```python
from build123d import *

# Parameters (mm, degrees)
CHANFREIN1_SIZE         = 0.5
CHANFREIN2_SIZE         = 1
ESQUISSE2_W             = 9
ESQUISSE2_H             = 30
ENL_V_MAT_EXTRU_1_DEPTH = 30
ENL_V_MAT_EXTRU_2_REACH = 84.195
ESQUISSE3_R             = 4.1
CHANFREIN3_SIZE         = 0.5
ENL_V_MAT_EXTRU_3_REACH = 53.962
ESQUISSE5_W             = 20
ESQUISSE5_H             = 3.5


with BuildPart() as part:
    # Esquisse1 → Révolution1 (revolve)
    with BuildSketch(Plane.XY, mode=Mode.PRIVATE) as r_volution1_sk:
        Polygon((-50, 8), (-65, 8), (-65, 5), (-66, 5), (-66, 6), (-80, 6), (-80, 0), (0, 0), (0, 10), (-50, 10), align=None)
    revolve(r_volution1_sk.sketch.rotate(Axis((0, 0, 0), (1, 0, 0)), 90), axis=Axis((0, 0, 0), (1, 0, 0)))

    # Chanfrein1
    chanfrein1_edges = [part.edges().sort_by_distance(p)[0] for p in [
        (-50, 0, -10),
        (0, 0, -10),
        (-65, 0, -8),
    ]]
    chamfer(chanfrein1_edges, length=CHANFREIN1_SIZE)

    # Chanfrein2
    chanfrein2_edges = [part.edges().sort_by_distance(p)[0] for p in [
        (-80, 0, -6),
    ]]
    chamfer(chanfrein2_edges, length=CHANFREIN2_SIZE)

    # Esquisse2 → Enlèv. mat.-Extru.1 (cut)
    with BuildSketch(Plane(origin=(0, 0, 0), x_dir=(0, 0, -1), z_dir=(1, 0, 0))):
        with Locations((-10.5, 0)):
            Rectangle(ESQUISSE2_W, ESQUISSE2_H)
        with Locations((10.5, 0)):
            Rectangle(ESQUISSE2_W, ESQUISSE2_H)
    extrude(amount=-ENL_V_MAT_EXTRU_1_DEPTH, mode=Mode.SUBTRACT)

    # Esquisse3 → Enlèv. mat.-Extru.2 (cut, up to next)
    with BuildSketch(Plane.XY.offset(6), mode=Mode.PRIVATE) as enl_v_mat_extru_2_sk1:
        with Locations((-11.5, 0)):
            Circle(ESQUISSE3_R)
    enl_v_mat_extru_2_tool1 = extrude(enl_v_mat_extru_2_sk1.sketch, amount=-ENL_V_MAT_EXTRU_2_REACH, mode=Mode.PRIVATE) & part.part
    add(enl_v_mat_extru_2_tool1.solids().sort_by_distance((-11.5, 0, 6))[0], mode=Mode.SUBTRACT)

    # Chanfrein3
    chanfrein3_edges = [part.edges().sort_by_distance(p)[0] for p in [
        (-15.6, 0, 6),
        (-15.6, 0, -6),
    ]]
    chamfer(chanfrein3_edges, length=CHANFREIN3_SIZE)

    # Esquisse5 → Enlèv. mat.-Extru.3 (cut, up to next)
    with BuildSketch(Plane.ZY.offset(50), mode=Mode.PRIVATE) as enl_v_mat_extru_3_sk1:
        with Locations((0, 8.25)):
            Rectangle(ESQUISSE5_W, ESQUISSE5_H)
    enl_v_mat_extru_3_tool1 = extrude(enl_v_mat_extru_3_sk1.sketch, amount=ENL_V_MAT_EXTRU_3_REACH, mode=Mode.PRIVATE) & part.part
    # Esquisse5 → Enlèv. mat.-Extru.3 (cut, up to next)
    with BuildSketch(Plane.ZY.offset(50), mode=Mode.PRIVATE) as enl_v_mat_extru_3_sk2:
        with Locations((0, -8.25)):
            Rectangle(ESQUISSE5_W, ESQUISSE5_H)
    enl_v_mat_extru_3_tool2 = extrude(enl_v_mat_extru_3_sk2.sketch, amount=ENL_V_MAT_EXTRU_3_REACH, mode=Mode.PRIVATE) & part.part
    add(enl_v_mat_extru_3_tool1.solids().sort_by_distance((-50, 8.25, 0))[0], mode=Mode.SUBTRACT)
    add(enl_v_mat_extru_3_tool2.solids().sort_by_distance((-50, -8.25, 0))[0], mode=Mode.SUBTRACT)


solid = part.part
```
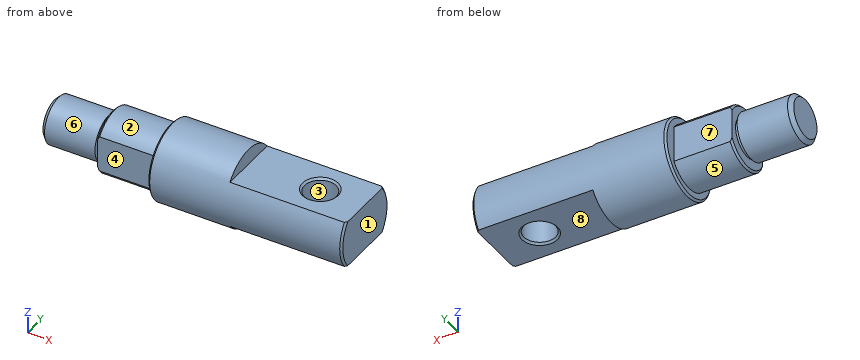
Source: CAD feature listing. Evaluate the final solid. Frame: model axes, mm. Face numbers are marked on the shaded views. A direction names the side the tool comes from. Round coordinates to 2 decimals unless told otherwise and drop trailing zeros. Loops run counter-clockwise (first coordinate to the right, second up) from the corner with the lowest first, then second, coordinate; pieces in that order, holes last. Notation, with made-up numbers: M 40,20.5 L 75,20.5 A30 cw 75,43.5 Z; hole C 59.5,-4 d4. An arc over 180 degrees is marked long. Use a Markdown table: item, result. Add a question column.
1. Line query: line 1 (X direction, y = 3.5, z = -4); line 2 (Y direction, x = -11.5, z = 0); line 3 (Y direction, x = -11.5, z = 1). Output: solid intervals per line, ascending.
2. Section query B-B on x = -11.5. Return the cut outline in (y, z), then the cut area to 3 significant figures.
3. Section query D-D on x = -55. Return the cut outline in (y, z), then the cut area to 3 significant figures.
4. Contact query for flat-ended pins moving along their axis: P1, Ø5, axis at x = -13.5, y = 1, coming from the -Z side; P2, Ø2, axis at y = 3.5, z = -8.5, coming from the +X side; P3, Ø3, axis at x = -24, y = 7, coming from the +Z side. Output: stop coordinate, or through.
5. Section query C-C on z = 0. Return the cut outline in (x, y), then the cut area to 3 significant figures.
6. Reachability of the marked faces 5, 6, 7 and 8 from +Z, -Z, +X, -X, +Y, -Y: full face, straight path, thin tool, end or side. Return the list, or none.
7. Mould query, pull axis Y, two halves, no side actions, for the marked faces 1, 2, 3 and 4. Classes: pulls with the +Y half, pulls with the -Y half, needs draft (parallel to the pull), parting line crosses it, or undercut.
Reported:
| question | item | result |
|---|---|---|
| 1 | line 1 | x = -79.68 to -66, -65 to -13.64, -9.36 to 0 |
| 1 | line 2 | y = -10 to -4.1, 4.1 to 10 |
| 1 | line 3 | y = -9.95 to -4.1, 4.1 to 9.95 |
| 2 | outline | M -8,-6 L -4.6,-6 L -4.1,-5.5 L -4.1,5.5 L -4.6,6 L -8,6 A10 ccw Z; M 4.1,-5.5 L 4.6,-6 L 8,-6 A10 ccw 8,6 L 4.6,6 L 4.1,5.5 Z |
| 2 | area | 126 mm² |
| 3 | outline | M -6.5,-4.66 A8 ccw 6.5,-4.66 L 6.5,4.66 A8 ccw -6.5,4.66 Z |
| 3 | area | 182 mm² |
| 4 | P1 | stops at z = -6 |
| 4 | P2 | stops at x = -30 |
| 4 | P3 | stops at z = 6 |
| 5 | outline | M -80,-5 L -79,-6 L -66,-6 L -66,-5 L -65,-5 L -65,-6.5 L -50,-6.5 L -50,-9.5 L -49.5,-10 L -0.5,-10 L 0,-9.5 L 0,9.5 L -0.5,10 L -49.5,10 L -50,9.5 L -50,6.5 L -65,6.5 L -65,5 L -66,5 L -66,6 L -79,6 L -80,5 Z; hole C -11.5,0 d8.2 |
| 5 | area | 1,320 mm² |
| 6 | face 5 | -Z, -X |
| 6 | face 6 | -X |
| 6 | face 7 | +Z, -Z, -X, +Y |
| 6 | face 8 | -Z, +X, +Y, -Y |
| 7 | face 1 | needs draft |
| 7 | face 2 | parting line crosses it |
| 7 | face 3 | undercut |
| 7 | face 4 | pulls with the -Y half |
